```python
from build123d import *

# Parameters (mm, degrees)
CYLINDER017_R     = 0.5
CYLINDER017_DEPTH = 20
CYLINDER018_R     = 0.5
CYLINDER018_DEPTH = 20
CYLINDER008_R     = 5
CYLINDER008_DEPTH = 13
PAD007_DEPTH      = 7
SKETCH065_W       = 2
SKETCH065_H       = 3
POCKET005_DEPTH   = 3


with BuildPart() as cylinder017:
    # Cylinder017 → Cylinder017 (new body)
    with BuildSketch(Plane(origin=(39, 12, 17.5), x_dir=(1, 0, 0), z_dir=(0, -1, 0))):
        Circle(CYLINDER017_R)
    extrude(amount=CYLINDER017_DEPTH)


with BuildPart() as fusion018:
    # Cylinder018 → Cylinder018 (new body)
    with BuildSketch(Plane(origin=(49, 12, 17.5), x_dir=(1, 0, 0), z_dir=(0, -1, 0))):
        Circle(CYLINDER018_R)
    extrude(amount=CYLINDER018_DEPTH)

    # Fusion018: union Cylinder017
    add(cylinder017.part)


with BuildPart() as cylinder008:
    # Cylinder008 → Cylinder008 (new body)
    with BuildSketch(Plane(origin=(56, -3, 21), x_dir=(1, 0, 0), z_dir=(0, 1, 0))):
        Circle(CYLINDER008_R)
    extrude(amount=CYLINDER008_DEPTH)


with BuildPart() as potclamp:
    # Sketch059 → Pad007 (new body)
    with BuildSketch(Plane.XY):
        with BuildLine():
            ThreePointArc((46.408643, 2.758552), (43.908643, 5.259517), (41.408643, 2.758552))
            Line((34.911109, 2.762902), (41.408643, 2.758552))
            ThreePointArc((52.911107, 2.762902), (43.911108, 11.758552), (34.911109, 2.762902))
            Line((46.408643, 2.758552), (52.911107, 2.762902))
        make_face()
    extrude(amount=PAD007_DEPTH)

    # Sketch065 → Pocket005 (cut)
    with BuildSketch(Plane.XY):
        with Locations((35.911109, 2.762661)):
            Rectangle(SKETCH065_W, SKETCH065_H)
    extrude(amount=POCKET005_DEPTH, mode=Mode.SUBTRACT)


with BuildPart() as potclamp_1:
    # Body007 placement: moved
    add(potclamp.part.moved(Location((0, 0, 14))))

    # Cut005: cut Cylinder008
    add(cylinder008.part, mode=Mode.SUBTRACT)

    # Cut011: cut Fusion018
    add(fusion018.part, mode=Mode.SUBTRACT)


solid = potclamp_1.part
```
Build history of the part. All positions in model axes, mm. A direction names the side the tool comes from. Round coordinates to 2 decimals unless told otherwise and drop trailing zeros. Write each loop counter-clockwise with the first axis right and the second up, starting at its lowest first coordinate (ties: lowest second). Pieces come first, ordered by that corner, then holes. Notation, with made-up numbers: (76.25, 57) - (125.25, 57) arc R13 cw to (125.25, 61) - close; hole circle Ø6 at (-20.75, -26). An arc over 180 degrees is marked (long way). Answer as CSV lines item,"result".
Q1. Pull direction Z, two halves, no side cores. Call faces 1 (the cylindrical face through (49, 7, 18)), 2 (the flat face through (44, 7, 14)), 3 (the flat face through (36, 4.263, 15)): +Z half, -Z half, draft (parallel to the pull), parting line (faces both ways), or undercut.
Report:
face 1,"undercut"
face 2,"-Z half"
face 3,"draft"
Q2. Cut at D-D (y = 6). Write the cut outline in (x, z), and give its area (3 significant figures).
Report:
outline,"(35.52, 14) - (52.31, 14) - (52.31, 17.63) arc R5 cw to (51, 21) - (35.52, 21) - close; hole circle Ø1 at (39, 17.5); hole circle Ø1 at (49, 17.5)"
area,"113 mm^2"
Q3. Tool access for faces 4 (the flat face through (36.911, 4, 15)), 5 (the flat face through (43, 7, 21)): list every direction of +Z, -Z, +X, -X, +Y, -Y with a clear straight run to the whole face (end or side of a thin tool).
Report:
face 4,"-Z, -X, -Y"
face 5,"+Z, +X, -X, +Y, -Y"
Q4. Drill centre lines: probe 1 along Z at (x, y) = (39, 5.75); probe 2 along X at (y, z) = (8.75, 17.5); probe 3 along X at (y, z) = (5.5, 17.5). Where is each one in solid material? Low to high. Write a range as [from, to].
Report:
probe 1,"z = [14, 17], [18, 21]"
probe 2,"x = [37.2, 38.5], [39.5, 48.5], [49.5, 50.63]"
probe 3,"x = [35.34, 38.5], [39.5, 48.5], [49.5, 52.43]"
Q5. Drop flat-ended pins along their axis: pin 1 (1.7 mm diameter, centred on x = 35.5, y = 3.5, fed in from -Z); pin 2 (1 mm diameter, centred on y = 8.5, z = 16, fed in from -X); pin 3 (1.5 mm diameter, centred on y = 4, z = 17.5, fed in from -X); pin 4 (1.5 mm diameter, centred on y = 8.5, z = 17.5, fed in from +X). Give the stop position or say it passes through.
Report:
pin 1,"stops at z = 14"
pin 2,"stops at x = 36.59"
pin 3,"stops at x = 34.92"
pin 4,"stops at x = 51.4"
Q6. Cut at C-C (z = 17.5). Write the cut outline in (x, y), and give its area (3 significant figures).
Report:
outline,"(34.91, 2.76) - (38.5, 2.76) - (38.5, 9.95) arc R9 ccw to start; (39.5, 2.76) - (41.41, 2.76) arc R2.5 cw to (46.41, 2.76) - (48.5, 2.76) - (48.5, 10.5) arc R9 ccw to (39.5, 10.6) - close; (49.5, 2.76) - (52.43, 2.76) - (52.43, 5.66) arc R9 ccw to (49.5, 9.81) - close"
area,"102 mm^2"
Q7. Cut at A-A (y = 5). Write the cut outline in (x, z), and give its area (3 significant figures).
Report:
outline,"(35.19, 14) - (42.8, 14) - (42.8, 21) - (35.19, 21) - close; (45.02, 14) - (52.63, 14) - (52.63, 17.31) arc R5 cw to (51, 21) - (45.02, 21) - close; hole circle Ø1 at (39, 17.5); hole circle Ø1 at (49, 17.5)"
area,"101 mm^2"
Q8. Cut at B-B (x = 39). Write the cut outline in (y, z), and give its area (3 significant figures).
Report:
outline,"(2.76, 14) - (10.3, 14) - (10.3, 17) - (2.76, 17) - close; (2.76, 18) - (10.3, 18) - (10.3, 21) - (2.76, 21) - close"
area,"45.2 mm^2"
